```python
from build123d import *

# Parameters (mm, degrees)
SKETCH1_W           = 25.4
SKETCH1_H           = 29.2862
BOSS_EXTRUDE1_DEPTH = 16.002
CUT_EXTRUDE1_DEPTH  = 5.842
SKETCH3_R           = 1.905
CUT_EXTRUDE2_DEPTH  = 80.18158073
CUT_EXTRUDE3_DEPTH  = 81.01960028


with BuildPart() as part:
    # Sketch1 → Boss-Extrude1 (new body)
    with BuildSketch(Plane.XY):
        with Locations((-60.028198895, -14.972879006)):
            Rectangle(SKETCH1_W, SKETCH1_H)
    extrude(amount=BOSS_EXTRUDE1_DEPTH)

    # Sketch2 → Cut-Extrude1 (cut)
    with BuildSketch(Plane.XY.offset(16.002)):
        with BuildLine():
            Line((-69.934198895, -9.508203302), (-69.934198895, -20.361354709))
            ThreePointArc((-69.934198895, -20.361354709), (-65.147057291, -27.422210503), (-65.362198895, -18.894249236))
            Line((-65.362198895, -18.894249236), (-65.362198895, -10.975308775))
            ThreePointArc((-65.362198895, -10.975308775), (-65.147057291, -2.447347508), (-69.934198895, -9.508203302))
        make_face()
    extrude(amount=-CUT_EXTRUDE1_DEPTH, mode=Mode.SUBTRACT)

    # Sketch3 → Cut-Extrude2 (cut, through all)
    with BuildSketch(Plane.XY.offset(10.16)):
        with Locations((-66.505198895, -6.679779006)):
            Circle(SKETCH3_R)
        with Locations((-66.505198895, -23.189779006)):
            Circle(SKETCH3_R)
    extrude(amount=-CUT_EXTRUDE2_DEPTH, mode=Mode.SUBTRACT)

    # Sketch4 → Cut-Extrude3 (cut, through all)
    with BuildSketch(Plane(origin=(0, -0.329779006, 0), x_dir=(1, 0, 0), z_dir=(0, 1, 0))):
        with BuildLine():
            Line((-57.488198895, -16.002), (-57.488198895, -14.166524863))
            ThreePointArc((-57.488198895, -14.166524863), (-59.057296313, -4.63042217), (-52.189613836, -11.43))
            Line((-52.189613836, -11.43), (-47.328198895, -11.43))
            Line((-47.328198895, -11.43), (-47.328198895, -16.002))
            Line((-47.328198895, -16.002), (-57.488198895, -16.002))
        make_face()
    extrude(amount=-CUT_EXTRUDE3_DEPTH, mode=Mode.SUBTRACT)


solid = part.part
```
Model file for the job. Use its own axes, mm. A direction names the side the tool comes from. Round coordinates to 2 decimals unless told otherwise and drop trailing zeros. Loops run counter-clockwise (first coordinate to the right, second up) from the corner with the lowest first, then second, coordinate; pieces in that order, holes last. Notation, with made-up numbers: M 82.5,48.25 L 108.5,48.25 A19 cw 108.5,85.25 Z; hole C 55,31.25 d2. An arc over 180 degrees is marked long. Put each result on its own line as item: value. Start each with the question number.
Item 1: Drop flat-ended pins along their axis: P1, Ø6, axis at x = -61, z = 11, coming from the +Y side; P2, Ø0.9, axis at y = -18, z = 14.5, coming from the +X side; P3, Ø5.5, axis at x = -66.51, y = -23.19, coming from the +Z side; P4, Ø4, axis at x = -51, y = -20, coming from the +Z side. Give the stop position or say it passes through.
Item 2: Cut at D-D (z = 13.25). List the corners of the cut face in (x, y) (3 decimals).
Item 3: Cut at A-A (z = 8). List the corners of the cut face in (x, y) (3 decimals), then the cut area to 3 significant figures.
Item 4: Cut at B-B (x = -59.75). List the corners of the cut face in (y, z), then the cut area to 3 significant figures.
Item 5: 3-axis set-ups, long thin cutter, end or side, ignore diameter. For faces 1 (the face through (-64.996, -2.499, 13.122)), 2 (the face through (-64, -15, 16.002)), 3 (the face through (-50, -15, 11.43)): which of +Z, -Z, +X, -X, +Y, -Y reach the whole face in a straight line?
Item 6: Cut at C-C (y = -18.5). List the corners of the cut face in (x, z), then the cut area to 3 significant figures.
Item 7: Mould opens along X. For faces 4 (the face through (-72.728, -15, 8)), 5 (the face through (-65.3, -27.47, 13.12)), 6 (the face through (-57.488, -15, 15)), 7 (the face through (-64.688, -6.108, 5.151)) say: released by +X, released by -X, zero draft, split by the parting line, or undercut.
Item 8: Drill centre lines: line 1 along Y through (x, z) = (-66.75, 8.5); line 2 along Y through (x, z) = (-70.5, 11); line 3 along X through (y, z) = (-4.25, 9). Where is each one in solid material? Low to high.
Answer block:
1. P1: y = -0.33
1. P2: x = -57.49
1. P3: z = 10.16
1. P4: z = 11.43
2. outline: M -72.728,-29.616 L -59.717,-29.616 L -59.717,-0.33 L -72.728,-0.33 Z; hole M -69.934,-20.361 A4.445 ccw long -65.362,-18.894 L -65.362,-10.975 A4.445 ccw long -69.934,-9.508 Z
3. outline: M -72.728,-29.616 L -61.676,-29.616 L -61.676,-0.33 L -72.728,-0.33 Z; M -51.777,-29.616 L -47.328,-29.616 L -47.328,-0.33 L -51.777,-0.33 Z; hole C -66.505,-23.19 d3.81; hole C -66.505,-6.68 d3.81
3. area: 431 mm2
4. outline: M -29.62,0 L -0.33,0 L -0.33,5.06 L -29.62,5.06 Z; M -29.62,13.23 L -0.33,13.23 L -0.33,16 L -29.62,16 Z
4. area: 230 mm2
5. face 1: +Z
5. face 2: +Z, +X, -X, +Y, -Y
5. face 3: +Z, +X, +Y, -Y
6. outline: M -72.73,0 L -47.33,0 L -47.33,11.43 L -52.19,11.43 A5.08 cw long -57.49,14.17 L -57.49,16 L -65.36,16 L -65.36,10.16 L -69.93,10.16 L -69.93,16 L -72.73,16 Z
6. area: 263 mm2
7. face 4: released by -X
7. face 5: undercut
7. face 6: released by +X
7. face 7: undercut
8. line 1: -29.62 to -25.08, -21.3 to -8.57, -4.79 to -0.33
8. line 2: -29.62 to -25.14, -21.24 to -8.63, -4.73 to -0.33
8. line 3: -72.73 to -61.8, -51.65 to -47.33
